Can you work these out from the model? Positions are in its coordinate system, mm. Round coordinates to 2 decimals unless told otherwise and drop trailing zeros. Loops run counter-clockwise (first coordinate to the right, second up) from the corner with the lowest first, then second, coordinate; pieces in that order, holes last.
```python
from build123d import *

# Parameters (mm, degrees)
F1_DEPTH = 100
F3_DEPTH = 45
F5_DEPTH = 30
F6_SIZE2 = 20
F6_SIZE  = 68
F8_DEPTH = 30
F9_SIZE2 = 22
F9_SIZE  = 88


with BuildPart() as f1:
    # F0 (on Front) → F1 (new body)
    with BuildSketch(Plane.XZ):
        Polygon((-22.5, 0), (0, 0), (0, 2007.5), (785, 2007.5), (785, 0), (807.5, 0), (807.5, 2030), (-22.5, 2030), align=None)
    extrude(amount=F1_DEPTH)

    # F2 (on face) → F3 (join)
    with BuildSketch(Plane(origin=(0, 0, 0), x_dir=(-1, 0, 0), z_dir=(0, 1, 0))):
        Polygon((12.5, 0), (22.5, 0), (32.5, 0), (32.5, 2040), (-817.5, 2040), (-817.5, 0), (-807.5, 0), (-797.5, 0), (-797.5, 2020), (12.5, 2020), align=None)
    extrude(amount=F3_DEPTH)

    # F4 (on face) → F5 (join)
    with BuildSketch(Plane(origin=(0, 45, 0), x_dir=(-1, 0, 0), z_dir=(0, 1, 0))):
        Polygon((-897.5, 0), (-817.5, 0), (-807.5, 0), (-807.5, 2035), (27.5, 2035), (27.5, 0), (32.5, 0), (112.5, 0), (112.5, 2120), (-897.5, 2120), align=None)
    extrude(amount=F5_DEPTH)

    # F6
    f6_edges = [f1.edges().sort_by_distance(p)[0] for p in [
        (390, 75, 2035),
        (-27.5, 75, 1017.5),
        (807.5, 75, 1017.5),
    ]]
    f6_side = f1.faces().sort_by_distance((852.5, 75, 23.482973))[0]
    chamfer(f6_edges, length=F6_SIZE, length2=F6_SIZE2, reference=f6_side)

    # F7 (on face) → F8 (join)
    with BuildSketch(Plane.XZ.offset(100)):
        Polygon((-118, 0), (-8, 0), (-8, 2015.5), (793, 2015.5), (793, 0), (903, 0), (903, 2125.5), (-118, 2125.5), align=None)
    extrude(amount=F8_DEPTH)

    # F9
    f9_edges = [f1.edges().sort_by_distance(p)[0] for p in [
        (793, -130, 1007.75),
        (392.5, -130, 2015.5),
        (-8, -130, 1007.75),
    ]]
    f9_side = f1.faces().sort_by_distance((-63, -130, 23.580058))[0]
    chamfer(f9_edges, length=F9_SIZE, length2=F9_SIZE2, reference=f9_side)


solid = f1.part
```
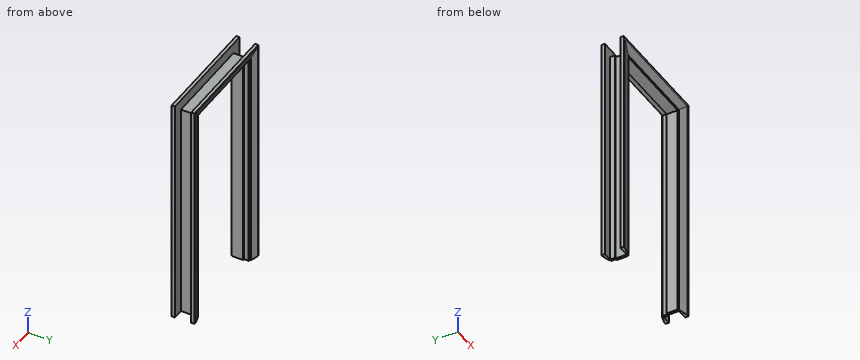
(1) Suppose I cut it at C-C (x = 450). Write out the boundary of the cut face in (y, z), then the cut area to 3 significant figures.
(2) Suppose I cut it at A-A (x = 839). Write out the boundary of the cut face in (y, z), then the cut area to 3 significant figures.
(3) If I drill on line 1 (X direction, y = -96.5, z = 1878); line 2 (X direction, y = 52, z = 1892.5); line 3 (Z direction, x = 307.5, y = -71.5), over which ranges is the centre line in solid material (lowest first)?
(4) For pin 1 (6 mm diameter, centred on x = 779.5, z = 1883, fed in from +Y); pin 2 (6.5 mm diameter, centred on x = 222, y = -105.5, fed in from -Z); pin 3 (11 mm diameter, centred on y = 48, z = 1422.5, fed in from -X); pin 4 (9 mm diameter, centred on x = 377, y = 66.5, fed in from +Z), each with a flat end and sliding along its axis, tell me the tip position at first contact or that it passes through.
(5) Suppose I cut it at B-B (y = 23). Write out the boundary of the cut face in (x, z).
Check result:
1. outline: (-130, 2103.5) - (-108, 2015.5) - (-100, 2015.5) - (-100, 2007.5) - (0, 2007.5) - (0, 2020) - (45, 2020) - (45, 2035) - (55, 2035) - (75, 2103) - (75, 2120) - (45, 2120) - (45, 2040) - (0, 2040) - (0, 2030) - (-100, 2030) - (-100, 2125.5) - (-130, 2125.5) - close
1. area: 7,350 mm2
2. outline: (-130, 2103.5) - (-119.5, 2061.5) - (-119.5, 0) - (-100, 0) - (-100, 2125.5) - (-130, 2125.5) - close; (45, 0) - (64.26, 0) - (64.26, 2066.5) - (75, 2103) - (75, 2120) - (45, 2120) - close
2. area: 83,100 mm2
3. line 1: x = -22.5 to 0, 785 to 807.5
3. line 2: x = -112.5 to -27.5, 807.5 to 897.5
3. line 3: z = 2007.5 to 2030
4. pin 1: passes through
4. pin 2: stops at z = 2015.5
4. pin 3: stops at x = -112.5
4. pin 4: stops at z = 2120
5. outline: (-32.5, 0) - (-12.5, 0) - (-12.5, 2020) - (797.5, 2020) - (797.5, 0) - (817.5, 0) - (817.5, 2040) - (-32.5, 2040) - close
